Verification items for the finished model (mm, model axes). A direction names the side the tool comes from. Give positions to 0.01 mm unless a question says otherwise; leave off trailing zeros. Loops run counter-clockwise (first coordinate to the right, second up) from the corner with the lowest first, then second, coordinate; pieces in that order, holes last. Notation, with made-up numbers: (-2.75, 70) - (13.25, 70) arc R11 cw to (13.25, 74) - close; hole circle Ø3 at (47, 13.5). An arc over 180 degrees is marked (long way). One line per question, with ' | ' between items. Start each with the question number.
1. Depth check by flat-ended pin: pin 1 Ø3 at (x, z) = (-43.9, 0) entering from +Y; pin 2 Ø3.5 at (x, z) = (18.1, -55) entering from -Y; pin 3 Ø5 at (x, z) = (-1.9, 75) entering from -Y; pin 4 Ø1 at (x, y) = (19.5, 1.5) entering from +Z. Enter the tip coordinate at first touch or a pass-through.
2. Tool access check on faces 1 (the face through (-47.38, 2, -21)), 2 (the face through (4, 1, 71)). Record the directions out of +Z, -Z, +X, -X, +Y, -Y that give a thin tool (end or side, any length) a straight path to the whole face; none if there is none.
3. Section check B-B, the plane x = -16. Enter the section's corners in (y, z).
4. Section check D-D, the plane z = 26.5. Enter the section's corners in (x, y), then the cut area to 3 significant figures.
5. Section check A-A, the plane z = -18.5. Enter the section's corners in (x, y), then the cut area to 3 significant figures.
6. Section check C-C, the plane y = 0.5. State how many separate pieces and enclosed holes the cut face has, then the cut area to 3 significant figures.
7. Thickness scan on line 1 along Z through (x, y) = (-6, 2.7); line 2 along X through (y, z) = (2.2, -55); line 3 along Z through (x, y) = (5, 1.35). Record the ranges inside material, lowest first. Write a range as from..to.
from build123d import *

# Parameters (mm, degrees)
SKETCH_1_W          = 160
SKETCH_1_H          = 136
SKETCH_1_R          = 40.9
SKETCH_1_R_2        = 1.55
SKETCH_1_R_3        = 1.6
EXTRUDE_1_DEPTH     = 3
SKETCH_2_W          = 25
SKETCH_2_H          = 136
EXTRUDE_2_DEPTH     = 3
SKETCH_3_W          = 90
SKETCH_3_H          = 136
CUT_EXTRUDE_1_DEPTH = 4
CUT_EXTRUDE_3_DEPTH = 4
FILLET_1_R          = 5
FILLET_2_R          = 5
CHAMFER_1_SIZE      = 1


with BuildPart() as part:
    # 草图1 → 凸台-拉伸1 (new body)
    with BuildSketch(Plane(origin=(0, 0, 0), x_dir=(1, 0, 0), z_dir=(0, 1, 0))):
        with Locations((-32.38, -10)):
            Rectangle(SKETCH_1_W, SKETCH_1_H)
        Circle(SKETCH_1_R, mode=Mode.SUBTRACT)
        with Locations((0, 43.9)):
            Circle(SKETCH_1_R_2, mode=Mode.SUBTRACT)
        with Locations((43.9, 0)):
            Circle(SKETCH_1_R_2, mode=Mode.SUBTRACT)
        with Locations((0, -43.9)):
            Circle(SKETCH_1_R_2, mode=Mode.SUBTRACT)
        with Locations((-43.9, 0)):
            Circle(SKETCH_1_R_2, mode=Mode.SUBTRACT)
        with Locations((-19.9, 39.130550724)):
            Circle(SKETCH_1_R_2, mode=Mode.SUBTRACT)
        with Locations((18.1, 55)):
            Circle(SKETCH_1_R_3, mode=Mode.SUBTRACT)
        with Locations((-1.9, 55)):
            Circle(SKETCH_1_R_3, mode=Mode.SUBTRACT)
        with Locations((-21.9, 55)):
            Circle(SKETCH_1_R_3, mode=Mode.SUBTRACT)
        with Locations((-41.9, 55)):
            Circle(SKETCH_1_R_3, mode=Mode.SUBTRACT)
        with Locations((18.1, -75)):
            Circle(SKETCH_1_R_3, mode=Mode.SUBTRACT)
        with Locations((-1.9, -75)):
            Circle(SKETCH_1_R_3, mode=Mode.SUBTRACT)
        with Locations((-21.9, -75)):
            Circle(SKETCH_1_R_3, mode=Mode.SUBTRACT)
        with Locations((-41.9, -75)):
            Circle(SKETCH_1_R_3, mode=Mode.SUBTRACT)
    extrude(amount=EXTRUDE_1_DEPTH)

    # 草图2 → 凸台-拉伸2 (add)
    with BuildSketch(Plane(origin=(0, 0, 0), x_dir=(1, 0, 0), z_dir=(0, 1, 0))):
        with Locations((-124.88, -10)):
            Rectangle(SKETCH_2_W, SKETCH_2_H)
    extrude(amount=EXTRUDE_2_DEPTH)

    # 草图3 → 切除-拉伸1 (cut, through all)
    with BuildSketch(Plane(origin=(0, 3, 0), x_dir=(1, 0, 0), z_dir=(0, 1, 0))):
        with Locations((-92.38, -10)):
            Rectangle(SKETCH_3_W, SKETCH_3_H)
    extrude(amount=-CUT_EXTRUDE_1_DEPTH, mode=Mode.SUBTRACT)

    # 草图4 → 切除-拉伸3 (cut, through all)
    with BuildSketch(Plane(origin=(0, 0, 0), x_dir=(1, 0, 0), z_dir=(0, 1, 0))):
        Polygon((47.62, 58), (47.62, 3.843146871), (22.215512532, 58), align=None)
        Polygon((47.62, -1.482721699), (47.62, -78), (21.298056264, -78), align=None)
        with BuildLine():
            Line((-20.395912494, -65.916645202), (-29.90797954, -33.48914391))
            ThreePointArc((-29.90797954, -33.48914391), (-18.489584756, -40.916320162), (-5.369508319, -44.577778998))
            Line((-5.369508319, -44.577778998), (-20.395912494, -65.916645202))
        make_face()
        with BuildLine():
            Line((-14.191049882, -71), (1.385146854, -48.880378151))
            ThreePointArc((1.385146854, -48.880378151), (13.780479279, -46.918103018), (25.268173443, -41.865611316))
            Line((25.268173443, -41.865611316), (15.245943736, -71))
            Line((15.245943736, -71), (-14.191049882, -71))
        make_face()
        Polygon((-47.38, -78), (-47.38, -26), (-47.38, -10), (-27.38, -78), align=None)
    extrude(amount=CUT_EXTRUDE_3_DEPTH, mode=Mode.SUBTRACT)

    # 圆角1
    fillet_1_edges = [part.edges().sort_by_distance(p)[0] for p in [
        (22.215512532, 1.5, -58),
        (47.62, 1.5, -3.843146871),
        (-27.38, 1.5, 78),
        (-47.38, 1.5, 10),
        (47.62, 1.5, 1.482721699),
        (21.298056264, 1.5, 78),
        (-47.38, 1.5, -58),
    ]]
    fillet(fillet_1_edges, radius=FILLET_1_R)

    # 圆角2
    fillet_2_edges = [part.edges().sort_by_distance(p)[0] for p in [
        (-14.191049882, 1.5, 71),
        (15.245943736, 1.5, 71),
        (25.268173443, 1.5, 41.865611316),
        (1.385146854, 1.5, 48.880378151),
        (-5.369508319, 1.5, 44.577778998),
        (-29.90797954, 1.5, 33.48914391),
        (-20.395912494, 1.5, 65.916645202),
    ]]
    fillet(fillet_2_edges, radius=FILLET_2_R)

    # 倒角1
    chamfer_1_edges = [part.edges().sort_by_distance(p)[0] for p in [
        (16.5, 0, -55),
        (-3.5, 0, -55),
        (-23.5, 0, -55),
        (-43.5, 0, -55),
        (16.5, 0, 75),
        (-3.5, 0, 75),
        (-23.5, 0, 75),
    ]]
    chamfer(chamfer_1_edges, length=CHAMFER_1_SIZE)


solid = part.part
Results list:
1) pin 1: through | pin 2: y = 0.85 | pin 3: y = 0.1 | pin 4: z = 77.84
2) face 1: +Z, -Z, -X, +Y, -Y | face 2: +Y, -Y
3) outline: (0, -58) - (3, -58) - (3, -37.64) - (0, -37.64) - close; (0, 37.64) - (3, 37.64) - (3, 41.95) - (0, 41.95) - close; (0, 58.88) - (3, 58.88) - (3, 78) - (0, 78) - close
4) outline: (-42.53, 0) - (-31.15, 0) - (-31.15, 3) - (-42.53, 3) - close; (31.15, 0) - (39.01, 0) - (39.01, 3) - (31.15, 3) - close | area: 57.7 mm²
5) outline: (-47.38, 0) - (-36.48, 0) - (-36.48, 3) - (-47.38, 3) - close; (36.48, 0) - (40.74, 0) - (40.74, 3) - (36.48, 3) - close | area: 45.5 mm²
6) separate pieces: 1 | enclosed holes: 15 | area: 4,340 mm²
7) line 1: -58..-40.46, 40.46..59.37, 70.79..78 | line 2: -46.96..-43.5, -40.3..-23.5, -20.3..-3.5, -0.3..16.5, 19.7..23.62 | line 3: -58..-40.59, 40.59..48.64, 71..78
